Could you check a few things on this model? Use its own coordinates, in mm. A direction names the side the tool comes from. Give positions to 0.01 mm unless a question says otherwise; leave off trailing zeros. Write each loop counter-clockwise with the first axis right and the second up, starting at its lowest first coordinate (ties: lowest second). Pieces come first, ordered by that corner, then holes. Notation, with made-up numbers: M -12,-21.75 L 17,-21.75 A26 cw 17,-1.75 Z; hole C -4.5,35 d8. An arc over 180 degrees is marked long. One line per item, written item: value.
```python
from build123d import *

# Parameters (mm, degrees)
ESQUISSE1_W                = 270
ESQUISSE1_H                = 270
EXTRUSION1_DEPTH           = 170
CONG_2_R                   = 4
EXTRUSION2_DEPTH           = 168
CONG_3_R                   = 4
TROU_TARAUD_4_481_D        = 2.3749
TROU_TARAUD_4_481_DEPTH    = 45
TROU_TARAUD_4_481_TIP      = 0.713491942
ESQUISSE5_W                = 14
ESQUISSE5_H                = 16
ENL_V_MAT_EXTRU_1_DEPTH    = 3
ESQUISSE6_R                = 6.75
ENL_V_MAT_EXTRU_6_DEPTH    = 10
R_P_TITION_LIN_AIRE3_COUNT = 4
R_P_TITION_LIN_AIRE3_PITCH = 20
ESQUISSE7_R                = 4.25
ENL_V_MAT_EXTRU_7_DEPTH    = 3
ESQUISSE8_R                = 2
ENL_V_MAT_EXTRU_8_DEPTH    = 171
ESQUISSE9_R                = 1
ENL_V_MAT_EXTRU_9_DEPTH    = 10
ESQUISSE10_W               = 19.2
ESQUISSE10_H               = 27
ENL_V_MAT_EXTRU_10_DEPTH   = 10
ESQUISSE11_R               = 5
ENL_V_MAT_EXTRU_11_DEPTH   = 10
ESQUISSE12_R               = 2
ENL_V_MAT_EXTRU_12_DEPTH   = 10


with BuildPart() as part:
    # Esquisse1 → Extrusion1 (new body)
    with BuildSketch(Plane.XY):
        with Locations((135, -135)):
            Rectangle(ESQUISSE1_W, ESQUISSE1_H)
    extrude(amount=EXTRUSION1_DEPTH)

    # Congé2
    cong_2_edges = [part.edges().sort_by_distance(p)[0] for p in [
        (0, 0, 85),
        (270, 0, 85),
        (270, -270, 85),
        (0, -270, 85),
    ]]
    fillet(cong_2_edges, radius=CONG_2_R)

    # Esquisse2 → Extrusion2 (cut)
    with BuildSketch(Plane.XY.offset(170)):
        Polygon((12, -2), (12, -19), (2, -19), (2, -251), (12, -251), (12, -268), (258, -268), (258, -251), (268, -251), (268, -19), (258, -19), (258, -2), align=None)
    extrude(amount=-EXTRUSION2_DEPTH, mode=Mode.SUBTRACT)

    # Congé3
    cong_3_edges = [part.edges().sort_by_distance(p)[0] for p in [
        (258, -19, 86),
        (258, -251, 86),
        (12, -251, 86),
        (12, -19, 86),
    ]]
    fillet(cong_3_edges, radius=CONG_3_R)

    # Trou taraudé #4-481
    with Locations(Plane(origin=(6, -6, 170), x_dir=(1, 0, 0), z_dir=(0, 0, 1))):
        with Locations((0, 0), (258, 0), (258, -258), (0, -258)):
            Hole(TROU_TARAUD_4_481_D / 2, depth=TROU_TARAUD_4_481_DEPTH)
            with Locations((0, 0, -(TROU_TARAUD_4_481_DEPTH + TROU_TARAUD_4_481_TIP / 2))):  # 118° drill point
                Cone(0, TROU_TARAUD_4_481_D / 2, TROU_TARAUD_4_481_TIP, mode=Mode.SUBTRACT)

    # Esquisse5 → Enlèv. mat.-Extru.1 (cut, through all)
    with BuildSketch(Plane(origin=(2, 0, 0), x_dir=(0, 0, -1), z_dir=(1, 0, 0))):
        with Locations((-40, -83.327995254)):
            Rectangle(ESQUISSE5_W, ESQUISSE5_H)
    extrude(amount=-ENL_V_MAT_EXTRU_1_DEPTH, mode=Mode.SUBTRACT)

    # Esquisse6 → Enlèv. mat.-Extru.6 (cut, symmetric)
    with BuildSketch(Plane(origin=(270, -440, 0), x_dir=(0, 0, -1), z_dir=(-1, 0, 0))):
        with Locations((-50, -400)):
            Circle(ESQUISSE6_R)
        with Locations((-30, -400)):
            Circle(ESQUISSE6_R)
    enl_v_mat_extru_6 = extrude(amount=ENL_V_MAT_EXTRU_6_DEPTH, both=True, mode=Mode.SUBTRACT)

    # Répétition linéaire3: Enlèv. mat.-Extru.6 ×4
    with Locations(*[(0, -i * R_P_TITION_LIN_AIRE3_PITCH, 0) for i in range(1, R_P_TITION_LIN_AIRE3_COUNT)]):
        add(enl_v_mat_extru_6, mode=Mode.SUBTRACT)

    # Esquisse7 → Enlèv. mat.-Extru.7 (cut)
    with BuildSketch(Plane(origin=(0, 0, 0), x_dir=(-1, 0, 0), z_dir=(0, 1, 0))):
        with Locations((-135, 46.2)):
            Circle(ESQUISSE7_R)
    extrude(amount=-ENL_V_MAT_EXTRU_7_DEPTH, mode=Mode.SUBTRACT)

    # Esquisse8 → Enlèv. mat.-Extru.8 (cut, through all)
    with BuildSketch(Plane(origin=(0, 0, 0), x_dir=(-1, 0, 0), z_dir=(0, 0, -1))):
        with Locations((-154.5, -50)):
            Circle(ESQUISSE8_R)
        with Locations((-115.5, -50)):
            Circle(ESQUISSE8_R)
        with Locations((-115.5, -90)):
            Circle(ESQUISSE8_R)
        with Locations((-154.5, -90)):
            Circle(ESQUISSE8_R)
    extrude(amount=-ENL_V_MAT_EXTRU_8_DEPTH, mode=Mode.SUBTRACT)

    # Esquisse9 → Enlèv. mat.-Extru.9 (cut)
    with BuildSketch(Plane(origin=(0, 0, 0), x_dir=(-1, 0, 0), z_dir=(0, 1, 0))):
        with Locations((-175, 30)):
            Circle(ESQUISSE9_R)
        with Locations((-166, 30)):
            Circle(ESQUISSE9_R)
        with Locations((-103, 30)):
            Circle(ESQUISSE9_R)
        with Locations((-94, 30)):
            Circle(ESQUISSE9_R)
    extrude(amount=-ENL_V_MAT_EXTRU_9_DEPTH, mode=Mode.SUBTRACT)

    # Esquisse10 → Enlèv. mat.-Extru.10 (cut)
    with BuildSketch(Plane(origin=(270, 0, 0), x_dir=(0, 0, -1), z_dir=(1, 0, 0))):
        with Locations((-39.6, -131.5)):
            Rectangle(ESQUISSE10_W, ESQUISSE10_H)
    extrude(amount=-ENL_V_MAT_EXTRU_10_DEPTH, mode=Mode.SUBTRACT)

    # Esquisse11 → Enlèv. mat.-Extru.11 (cut)
    with BuildSketch(Plane.XZ.offset(270)):
        with Locations((245, 10)):
            Circle(ESQUISSE11_R)
    extrude(amount=-ENL_V_MAT_EXTRU_11_DEPTH, mode=Mode.SUBTRACT)

    # Esquisse12 → Enlèv. mat.-Extru.12 (cut)
    with BuildSketch(Plane.XY.offset(2)):
        with Locations((82.5, -31.834379135)):
            Circle(ESQUISSE12_R)
        with Locations((5.5, -31.834379135)):
            Circle(ESQUISSE12_R)
        with Locations((5.192317745, -169.834379135)):
            Circle(ESQUISSE12_R)
        with Locations((82.5, -169.834379135)):
            Circle(ESQUISSE12_R)
    extrude(amount=-ENL_V_MAT_EXTRU_12_DEPTH, mode=Mode.SUBTRACT)


solid = part.part
```
1) On a 3-axis mill with a long thin cutter (end or side, diameter ignored), from which of +Z, -Z, +X, -X, +Y, -Y can I reach the whole of each face in a straight line? I mean faces 1 (the face through (133, -268, 87)), 2 (the face through (268.986, -60.297, 36.743)), 3 (the face through (249.77, -269.01, 11.5)). Say none if no direction works.
Outcome:
face 1: +Z
face 2: +X
face 3: -Y
2) If we section it at D-D, the plane y = -25: Write out the boundary of the cut face in (x, z), then the cut area to 3 significant figures.
Outcome:
outline: M 0,0 L 270,0 L 270,170 L 268,170 L 268,2 L 2,2 L 2,170 L 0,170 Z
area: 1,210 mm^2
3) If we section it at B-B, the plane y = -100: Write out the boundary of the cut face in (x, z).
Outcome:
outline: M 0,0 L 270,0 L 270,23.25 L 268,23.25 L 268,2 L 2,2 L 2,170 L 0,170 Z; M 268,36.75 L 270,36.75 L 270,43.25 L 268,43.25 Z; M 268,56.75 L 270,56.75 L 270,170 L 268,170 Z
4) If we section it at A-A, the plane y = -128.5: Write out the boundary of the cut face in (x, z).
Outcome:
outline: M 0,0 L 270,0 L 270,30 L 268,30 L 268,2 L 2,2 L 2,170 L 0,170 Z; M 268,49.2 L 270,49.2 L 270,170 L 268,170 Z
5) Please list where these lines run through material, in increasing order: L1, parallel to Z at x = 269.5, y = -80; L2, parallel to Y at x = 6, z = 155; L3, parallel to X at y = -264, z = 142. Write a range as from..to.
Outcome:
L1: z = 0..23.25, 36.75..43.25, 56.75..170
L2: y = -270..-265.19, -262.81..-251, -19..-7.19, -4.81..0
L3: x = 0..4.81, 7.19..12, 258..262.81, 265.19..270
6) If we section it at C-C, the plane z = 83.5: Write out the boundary of the cut face in (x, y), then the cut area to 3 significant figures.
Outcome:
outline: M 0,-266 A4 ccw 4,-270 L 266,-270 A4 ccw 270,-266 L 270,-4 A4 ccw 266,0 L 4,0 A4 ccw 0,-4 Z; hole M 2,-251 L 8,-251 A4 cw 12,-255 L 12,-268 L 258,-268 L 258,-255 A4 cw 262,-251 L 268,-251 L 268,-19 L 262,-19 A4 cw 258,-15 L 258,-2 L 12,-2 L 12,-15 A4 cw 8,-19 L 2,-19 Z
area: 2,800 mm^2
7) We'd pull the mould along Z, two halves only. Please class faces 4 (the face through (269.014, -60.297, 56.743)), 5 (the face through (133, -133, 0)), 6 (the face through (133, 0, 84)), 7 (the face through (138.132, -0.986, 49.072)): pulls with the +Z half, pulls with the -Z half, needs draft (parallel to the pull), parting line crosses it, or undercut.
Outcome:
face 4: undercut
face 5: pulls with the -Z half
face 6: needs draft
face 7: undercut
8) I'm going to push flat-ended pins straight in: pin 1 (5 mm diameter, centred on x = 55, y = -211.5, fed in from +Z); pin 2 (1.6 mm diameter, centred on x = 1.5, z = 37.5, fed in from +Y). Where does each tip first touch, or does it pass through?
Outcome:
pin 1: stops at z = 2
pin 2: stops at y = -0.38
